Study the drawing (mm; zero at the part's minimum x, y, z) and answer. A direction names the side the tool comes from. Round coordinates to 2 decimals unless told otherwise and drop trailing zeros. Order: outer loops, then holes, each group sorted by start corner. A loop starts at its lowest first (then second) coordinate and runs counter-clockwise, first axis right, second up. Notation, with made-up numbers: (24.25, -29) -> (29.25, -29) arc R22 ccw to (29.25, 10) -> close; hole circle Ø4 at (-30, 76). An arc over 180 degrees is marked (long way). Answer in a Markdown table with one row per item. Add a question column.
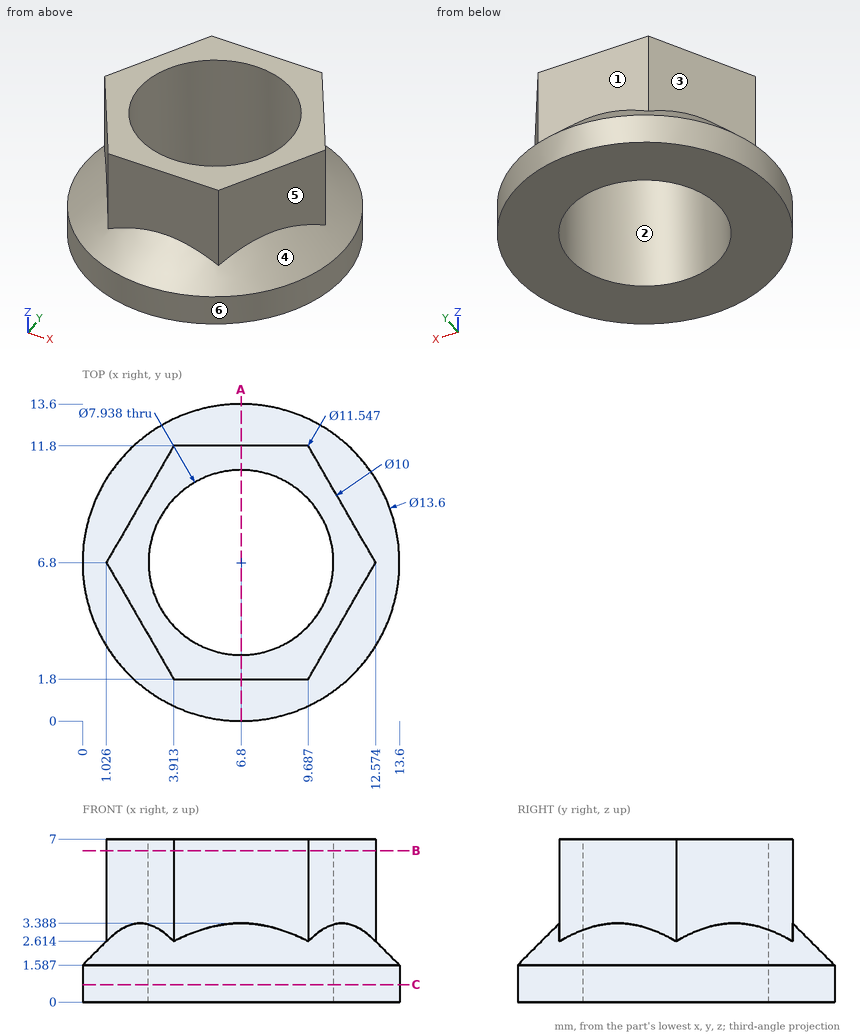
Item 1: A tool of negligible diameter and unlimited length cuts with its end or side. For the marked faces 5 and 6, from which of +Z, -Z, +X, -X, +Y, -Y can it reach the whole face along a straight path? Write none if from no direction.
Item 2: The part is cut by section A-A, the plane x = 6.8. Give the vertices of the cut face in (y, z), and give its area (3 significant figures).
Item 3: Flat-ended cylindrical pins translate along their axes: P1, Ø1, axis at y = 12, z = 6, coming from the +X side; P2, Ø4, axis at x = 2, z = 1, coming from the +Y side; P3, Ø3.5, axis at x = 6.5, z = 5.5, coming from the +Y side; P4, Ø6.5, axis at x = 6.8, y = 6.8, coming from the +Z side. Find the tip coordinate at first contact, or state that the pin passes through.
Item 4: The part is cut by section B-B, the plane z = 6.5. Give the vertices of the cut face in (x, y).
Item 5: Find the intervals of material crossed by probe 1 along Y at (x, z) = (6.8, 5); probe 2 along Y at (x, z) = (6.8, 1.5); probe 3 along X at (y, z) = (9, 1.5) (1 decimal), in increasing order. Write a range as [from, to].
Item 6: The part is cut by section C-C, the plane z = 0.75. Give the vertices of the cut face in (x, y).
Item 7: For a pull along X with two mould halves and no side action, classify the marked faces 1, 2, 3 and 4 as released by +X, released by -X, zero draft, split by the parting line, or undercut.
Resolved:
| question | item | result |
|---|---|---|
| 1 | face 5 | +Z, +X, -Y |
| 1 | face 6 | +Z, -Z |
| 2 | outline | (0, 0) -> (2.83, 0) -> (2.83, 7) -> (1.8, 7) -> (1.8, 3.39) -> (0, 1.59) -> close; (10.77, 0) -> (13.6, 0) -> (13.6, 1.59) -> (11.8, 3.39) -> (11.8, 7) -> (10.77, 7) -> close |
| 2 | area | 23.4 mm2 |
| 3 | P1 | x = 9.86 |
| 3 | P2 | y = 13 |
| 3 | P3 | y = 11.8 |
| 3 | P4 | through |
| 4 | outline | (1.03, 6.8) -> (3.91, 1.8) -> (9.69, 1.8) -> (12.57, 6.8) -> (9.69, 11.8) -> (3.91, 11.8) -> close; hole circle Ø7.94 at (6.8, 6.8) |
| 5 | probe 1 | [1.8, 2.83], [10.77, 11.8] |
| 5 | probe 2 | [0, 2.83], [10.77, 13.6] |
| 5 | probe 3 | [0.4, 3.5], [10.1, 13.2] |
| 6 | outline | circle Ø13.6 at (6.8, 6.8); hole circle Ø7.94 at (6.8, 6.8) |
| 7 | face 1 | zero draft |
| 7 | face 2 | undercut |
| 7 | face 3 | released by -X |
| 7 | face 4 | split by the parting line |
